Here's how the part is built. I have some questions about the finished solid (model axes, mm). A direction names the side the tool comes from. Give positions to 0.01 mm unless a question says otherwise; leave off trailing zeros. Order: outer loops, then holes, each group sorted by start corner. A loop starts at its lowest first (then second) coordinate and runs counter-clockwise, first axis right, second up. Notation, with made-up numbers: M 46,12.25 L 84,12.25 A20 ccw 84,39.25 Z; hole C -5.5,32.5 d3. An arc over 180 degrees is marked long. Use one line per item in the form item = value.
Autodesk Inventor part; units mm, degrees
ref_plane "YZ Plane" through (0, 0, 0) normal (1, 0, 0) x (0, 1, 0)
ref_plane "XZ Plane" through (0, 0, 0) normal (0, 1, 0) x (-1, 0, 0)
ref_plane "XY Plane" through (0, 0, 0) normal (0, 0, 1) x (1, 0, 0)
sketch "Sketch1" plane through (0, 0, 0) normal (0, 1, 0) x (-1, 0, 0)
  circle A0 centre (0, 0) radius 6
  dimension "d0" = 12
extrude "Extrusion1" add sketch "Sketch1" along normal blind 4
sketch "Sketch2" plane through (0, 4, 0) normal (0, 1, 0) x (1, 0, 0)
  circle A0 centre (0, 0) radius 4
  dimension "d3" = 8
extrude "Extrusion2" add sketch "Sketch2" along normal blind 10
sketch "Sketch3" plane through (0, 14, 0) normal (0, 1, 0) x (1, 0, 0)
  circle A0 centre (0, 0) radius 2
  dimension "d6" = 4
extrude "Extrusion3" cut sketch "Sketch3" against normal through all
chamfer "Chamfer1" distance 2 angle 45 1 edges at (-2, 0, 0)
properties part number "tube_long"
Q1. Thinking about a two-plate mould opening in Z: for faces 1 (the face through (0.98, 1.87, -1.89)), 2 (the face through (-2, 14, 1)), 3 (the face through (0, 8, 2)), 4 (the face through (6, 2, 0)), which applies, +Z half, -Z half, draft (parallel to the pull), parting line (faces both ways), or undercut?
Found:
face_1 = undercut
face_2 = draft
face_3 = undercut
face_4 = parting line
Q2. On a 3-axis mill with a long thin cutter (end or side, diameter ignored), from which of +Z, -Z, +X, -X, +Y, -Y can I reach the whole of each face in a straight line? I mean faces 5 (the face through (1.42, 0, -3.92)), 6 (the face through (1.42, 4, -3.92)). Say none if no direction works.
Found:
face_5 = +Z, -Z, +X, -X, -Y
face_6 = +Y
Q3. I want a section at B-B on x = 0. Write out the boundary of the cut face in (y, z).
Found:
outline = M 0,-6 L 4,-6 L 4,-4 L 14,-4 L 14,-2 L 2,-2 L 0,-4 Z; M 0,4 L 2,2 L 14,2 L 14,4 L 4,4 L 4,6 L 0,6 Z
Q4. I want a section at D-D on z = -5. Write out the boundary of the cut face in (x, y).
Found:
outline = M -3.32,0 L 3.32,0 L 3.32,4 L -3.32,4 Z
Q5. I want a section at C-C on y = 10.75. Write out the boundary of the cut face in (x, z).
Found:
outline = C 0,0 d8; hole C 0,0 d4
Q6. I want a section at A-A on z = 0. Write out the boundary of the cut face in (x, y), then the cut area to 3 significant figures.
Found:
outline = M -6,0 L -4,0 L -2,2 L -2,14 L -4,14 L -4,4 L -6,4 Z; M 2,2 L 4,0 L 6,0 L 6,4 L 4,4 L 4,14 L 2,14 Z
area = 68.0 mm²
Q7. I'm going to push flat-ended pins straight in: pin 1 Ø1.5 at (y, z) = (8, 4) entering from +X; pin 2 Ø4 at (x, z) = (4.5, 4.5) entering from +Y; pin 3 Ø3 at (x, y) = (-2.5, 7.5) entering from +Z. Where does each tip first touch, or does it pass through?
Found:
pin_1 = 2.33
pin_2 = 4
pin_3 = 3.87
Q8. I need wall thicknesses on L1, parallel to Z at x = 0, y = 6.5; L2, parallel to Y at x = -4, z = -0.5. Which ranges of each line are inside material? Lowest first, please.
Found:
L1 = -4 to -2, 2 to 4
L2 = 0 to 4
